```python
from build123d import *

# Parameters (mm, degrees)
ESQUISSE1_R        = 2.75
BOSS_EXTRU_1_DEPTH = 70


with BuildPart() as part:
    # Esquisse1 → Boss.-Extru.1 (new body)
    with BuildSketch(Plane(origin=(0, 0, 0), x_dir=(0, -1, 0), z_dir=(-1, 0, 0))):
        Polygon((-3, -10), (-3, -4.5), (3, -4.5), (3, -10), (10, -10), (10, -3), (4.5, -3), (4.5, 3), (10, 3), (10, 10), (3, 10), (3, 4.5), (-3, 4.5), (-3, 10), (-10, 10), (-10, 3), (-4.5, 3), (-4.5, -3), (-10, -3), (-10, -10), align=None)
        Circle(ESQUISSE1_R, mode=Mode.SUBTRACT)
    extrude(amount=-BOSS_EXTRU_1_DEPTH)


solid = part.part
```
Input: part model. Units: mm. Frame: model coordinates. A direction names the side the tool comes from. Give positions to 0.01 mm unless a question says otherwise; leave off trailing zeros. Order: outer loops, then holes, each group sorted by start corner. A loop starts at its lowest first (then second) coordinate and runs counter-clockwise, first axis right, second up.
1. Pin query (flat end, axial travel): pin 1 (3 mm diameter, centred on x = 21.5, y = -1, fed in from +Z); pin 2 (1.8 mm diameter, centred on x = 24, z = 1, fed in from -Y); pin 3 (3 mm diameter, centred on x = 36.5, z = 0, fed in from +Y). Return the tip coordinate at first contact, or that it passes through.
Derived:
pin 1: stops at z = 4.5
pin 2: stops at y = -4.5
pin 3: stops at y = 4.5
2. Mould query, pull axis Y, two halves, no side actions, for faces 4 (the flat face through (70, -2.1, -2.1)), 5 (the flat face through (35, 4.5, 0)), 6 (the flat face through (35, -4.5, 0)), 7 (the cylindrical face through (34.51, 0.596, -2.685)). Classes: released by +Y, released by -Y, zero draft, split by the parting line, or undercut.
Derived:
face 4: zero draft
face 5: released by +Y
face 6: released by -Y
face 7: undercut
3. Section A-A on z = -6.5. Return the cut outline in (x, y).
Derived:
outline: (0, -10) - (70, -10) - (70, -3) - (0, -3) - close; (0, 3) - (70, 3) - (70, 10) - (0, 10) - close
4. Material intervals for L1, parallel to Z at x = 54, y = 0; L2, parallel to Y at x = 41, z = 9.25, sorted ascending.
Derived:
L1: z = -4.5 to -2.75, 2.75 to 4.5
L2: y = -10 to -3, 3 to 10
5. Reachability of faces 1 (the flat face through (35, -3, 7)), 2 (the flat face through (35, -7, 3)), 3 (the flat face through (35, 7, 3)) from +Z, -Z, +X, -X, +Y, -Y: full face, straight path, thin tool, end or side. Return the list, or none.
Derived:
face 1: +Z, +X, -X
face 2: +X, -X, -Y
face 3: +X, -X, +Y
6. Section C-C on x = 35. Return the cut outline in (y, z), and give its area (3 significant figures).
Derived:
outline: (-10, -10) - (-3, -10) - (-3, -4.5) - (3, -4.5) - (3, -10) - (10, -10) - (10, -3) - (4.5, -3) - (4.5, 3) - (10, 3) - (10, 10) - (3, 10) - (3, 4.5) - (-3, 4.5) - (-3, 10) - (-10, 10) - (-10, 3) - (-4.5, 3) - (-4.5, -3) - (-10, -3) - close; hole circle Ø5.5 at (0, 0)
area: 244 mm2
7. Section B-B on y = 0. Return the cut outline in (x, z), and give its area (3 significant figures).
Derived:
outline: (0, -4.5) - (70, -4.5) - (70, -2.75) - (0, -2.75) - close; (0, 2.75) - (70, 2.75) - (70, 4.5) - (0, 4.5) - close
area: 245 mm2
